Solid Edge part; units mm, degrees
sketch "Sketch1" plane through (0, 0, 0) normal (0, 0, 1) x (1, 0, 0)
  circle A0 centre (0, 0) radius 95
extrude "Protrusion1" add sketch "Sketch1" against normal blind 5
sketch "Sketch2" plane through (0, 0, 0) normal (0, 0, 1) x (1, 0, 0)
  circle A0 centre (-2.5, 0) radius 1.5
  circle A1 centre (2.5, 0) radius 1.5
extrude "Wyciągnięcie_2" add sketch "Sketch2" along normal blind 15
sketch "Sketch3" plane through (0, 0, 0) normal (0, 0, 1) x (1, 0, 0)
  line L0 (-10, 60) -> (10, 60)
  line L1 (10, 60) -> (10, 70)
  line L2 (10, 70) -> (-10, 70)
  line L3 (-10, 70) -> (-10, 60)
extrude "Cutout1" cut sketch "Sketch3" against normal up to next
sketch "Sketch4" plane through (0, 60, -2.5) normal (0, 1, 0) x (0, 0, 1)
  circle A0 centre (0, 0) radius 1
extrude "Wyciągnięcie_4" add sketch "Sketch4" along normal blind 16
sketch "Sketch5" plane through (0, 62, -2.5) normal (0, 1, 0) x (0, 0, 1)
  circle A0 centre (0, 0) radius 4
extrude "Wyciągnięcie_5" add sketch "Sketch5" along normal blind 6
hole "Otwór_5" at (-63.6396, -63.6396, 0) direction (0, 0, -1) diameter 2.459 depth 11
sketch "Sketch6" plane through (0, 0, 0) normal (0, 0, 1) x (0, 1, 0)
  circle A0 centre (-63.6396, 63.6396) radius 2.5
extrude "Wycięcie_27" cut sketch "Sketch6" against normal blind 2.5
pattern_circular "Pattern1" count 4 over 360 about axis through (0, 0, 0) along (0, 0, -1) of "Wycięcie_27", "Otwór_5"
sketch "Sketch7" plane through (0, 95, -10) normal (0, 1, 0) x (0, 0, 1)
  circle A0 centre (7.5, 0) radius 1.5
extrude "Wyciągnięcie_19" add sketch "Sketch7" against normal blind 1.2757 and the other way blind 1
pattern_circular "Pattern3" count 4 over 360 about axis through (0, 0, 0) along (0, 0, 1) of "Wyciągnięcie_19"
pattern_circular "Pattern5" count 4 over 360 about axis through (0, 0, 0) along (0, 0, -1) of "Cutout1"
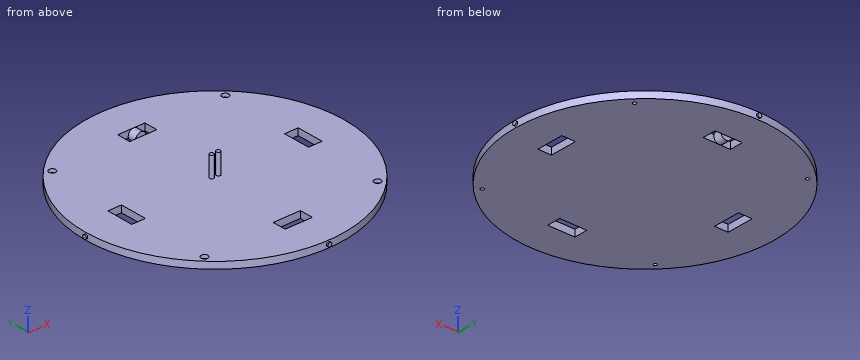
Geometry check sheet. Reference: the model listing, model coordinates, mm. Round coordinates to 2 decimals unless told otherwise and drop trailing zeros. Order: outer loops, then holes, each group sorted by start corner. A loop starts at its lowest first (then second) coordinate and runs counter-clockwise, first axis right, second up. Notation, with made-up numbers: M -27,55.25 L 4,55.25 A19 cw 4,88.25 Z; hole C -4.75,58 d8. An arc over 180 degrees is marked long. Write item = value, one per line.
Q1. Section check A-A (z = 4). Enter the section's corners in (x, y).
Answer block:
outline = C -2.5,0 d3; C 2.5,0 d3
Q2. Depth check by flat-ended pin: pin 1 Ø8 at (x, y) = (63.64, 63.64) entering from -Z; pin 2 Ø2.5 at (y, z) = (63.5, -2.5) entering from -X; pin 3 Ø5.5 at (y, z) = (-67, -1.5) entering from +X; pin 4 Ø2.5 at (y, z) = (-1.5, -3) entering from -X. Enter the tip coordinate at first touch or a pass-through.
Answer block:
pin_1 = -5
pin_2 = -71.76
pin_3 = 69.98
pin_4 = -96
Q3. Scan lines: line 1 (Z direction, x = -43, y = -14); line 2 (Y direction, x = 78.5, z = -0.75); line 3 (Y direction, x = -32.5, z = -3). Record each from-to range of solid material in increasing order.
Answer block:
line_1 = -5 to 0
line_2 = -53.5 to 53.5
line_3 = -89.27 to 89.27
Q4. Section check B-B (x = 56). Enter the section's corners in (y, z), plus the area to 3 significant figures.
Answer block:
outline = M -76.74,-5 L 76.74,-5 L 76.74,0 L -76.74,0 Z
area = 767 mm^2
Q5. Section check C-C (x = -56.5). Enter the section's corners in (y, z).
Answer block:
outline = M -76.37,-5 L 76.37,-5 L 76.37,0 L -76.37,0 Z
